Verification items for the finished model (mm, model axes). A direction names the side the tool comes from. Coordinates: 2 decimals unless noted, no trailing zeros. Order: outer loops, then holes, each group sorted by start corner. A loop starts at its lowest first (then second) coordinate and runs counter-clockwise, first axis right, second up. Notation, with made-up numbers: M 25,-7.75 L 57,-7.75 A15 ccw 57,18.25 Z; hole C 31,57.25 d10. An arc over 180 degrees is marked long. Return JSON: item names as keys, results as strings. Group by question number.
1. Section check D-D, the plane x = -6.5. Record the cut outline in (y, z), plus the area to 3 significant figures.
2. Section check B-B, the plane y = 0. Record the cut outline in (x, z), plus the area to 3 significant figures.
3. Section check C-C, the plane x = 20. Record the cut outline in (y, z), plus the area to 3 significant figures.
4. Section check A-A, the plane z = -15.25. Record the cut outline in (x, y), plus the area to 3 significant figures.
5. Set-up check for faces 1 (the cylindrical face through (-5.39, 16.01, -9.37)), 2 (the flat face through (23.586, 18.901, 1.972)): record each of +Z, -Z, +X, -X, +Y, -Y from which the full face is reachable in a straight line by a thin tool's end or side.
6. Material ranges on line 1 along Z through (x, y) = (-6.5, 12); line 2 along Y through (x, z) = (21, -10); line 3 along X through (y, z) = (0.5, -5), recorded low to high.
7. Gauge pin test, flat ends, axial feed: pin 1 (1 mm diameter, centred on x = 9.5, y = 3.5, fed in from -Z); pin 2 (1.5 mm diameter, centred on x = 19.5, z = -3.5, fed in from -Y); pin 3 (4 mm diameter, centred on y = -14.5, z = -15.5, fed in from -X); pin 4 (12 mm diameter, centred on x = 16, z = -1, fed in from -Y). Record the tip position at first contact, or that the pin passes through.
```python
from build123d import *

# Parameters (mm, degrees)
ESQUISSE1_W        = 42.15149663
ESQUISSE1_H        = 42.731591692
BOSS_EXTRU_1_DEPTH = 4
CHANFREIN1_SIZE    = 5
ESQUISSE3_R        = 1.5
BOSS_EXTRU_3_DEPTH = 19


with BuildPart() as part:
    # Esquisse1 → Boss.-Extru.1 (new body)
    with BuildSketch(Plane.XY):
        with Locations((5.045077825, 0)):
            Rectangle(ESQUISSE1_W, ESQUISSE1_H)
    extrude(amount=BOSS_EXTRU_1_DEPTH)

    # Chanfrein1
    chanfrein1_edges = [part.edges().sort_by_distance(p)[0] for p in [
        (-16.03067049, -21.365795846, 2),
        (-16.03067049, 21.365795846, 2),
        (26.12082614, 21.365795846, 2),
        (26.12082614, -21.365795846, 2),
    ]]
    chamfer(chanfrein1_edges, length=CHANFREIN1_SIZE)

    # Esquisse3 → Boss.-Extru.3 (add)
    with BuildSketch(Plane(origin=(0, 0, 0), x_dir=(-1, 0, 0), z_dir=(0, 0, -1))):
        with Locations((-20, 0)):
            Circle(ESQUISSE3_R)
        with Locations((6.5, 15)):
            Circle(ESQUISSE3_R)
        with Locations(Location((6.5, -15, 0), (0, 0, 180))):
            Circle(ESQUISSE3_R)
    extrude(amount=BOSS_EXTRU_3_DEPTH)


solid = part.part
```
Answers follow:
{
 "1": {"outline": "M -21.37,0 L -16.5,0 L -16.5,-19 L -13.5,-19 L -13.5,0 L 13.5,0 L 13.5,-19 L 16.5,-19 L 16.5,0 L 21.37,0 L 21.37,4 L -21.37,4 Z", "area": "285 mm^2"},
 "2": {"outline": "M -16.03,0 L 18.5,0 L 18.5,-19 L 21.5,-19 L 21.5,0 L 26.12,0 L 26.12,4 L -16.03,4 Z", "area": "226 mm^2"},
 "3": {"outline": "M -21.37,0 L -1.5,0 L -1.5,-19 L 1.5,-19 L 1.5,0 L 21.37,0 L 21.37,4 L -21.37,4 Z", "area": "228 mm^2"},
 "4": {"outline": "C -6.5,-15 d3; C -6.5,15 d3; C 20,0 d3", "area": "21.2 mm^2"},
 "5": {"face 1": "-Z", "face 2": "+Z, -Z, +X, +Y"},
 "6": {"line 1": "0 to 4", "line 2": "-1.12 to 1.12", "line 3": "18.59 to 21.41"},
 "7": {"pin 1": "z = 0", "pin 2": "y = -1.5", "pin 3": "x = -8", "pin 4": "y = -21.37"}
}
